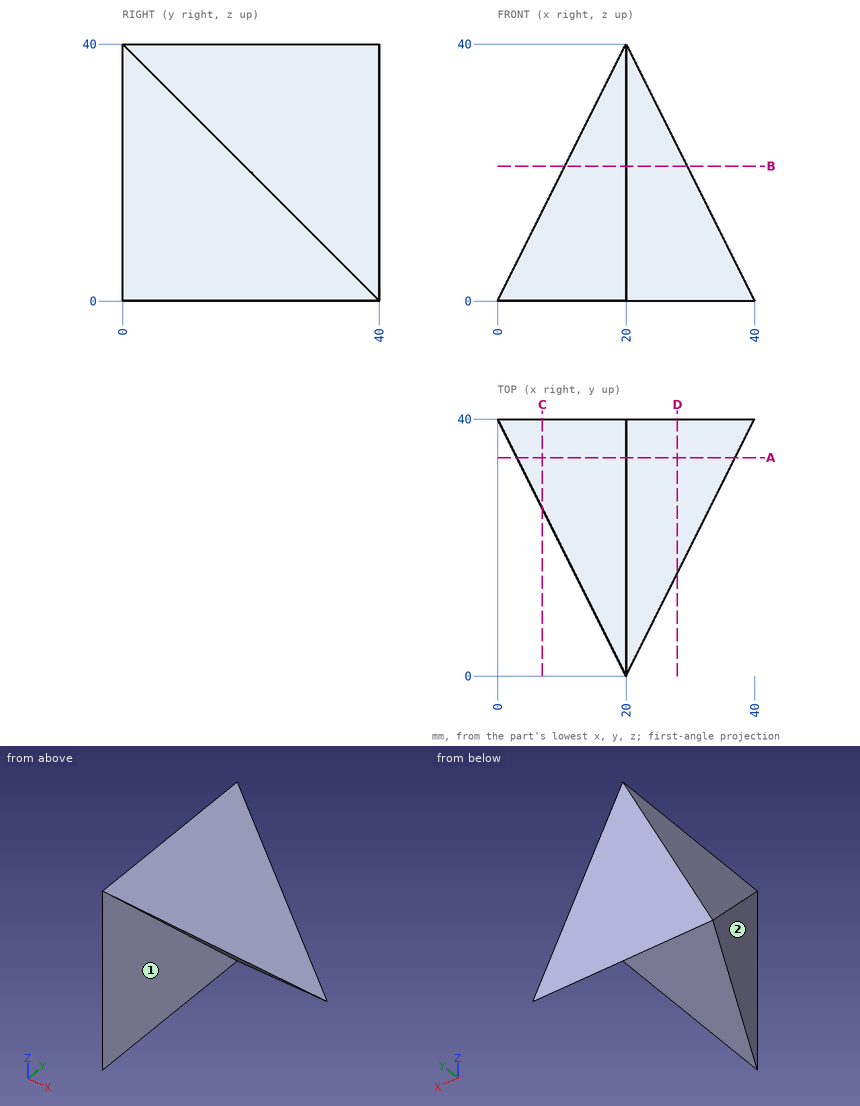
Print and shaded views of the part. All mm, measured from the part's lowest x, y and z. A direction names the side the tool comes from. Coordinates: 2 decimals unless noted, no trailing zeros. Order: outer loops, then holes, each group sorted by start corner. A loop starts at its lowest first (then second) coordinate and runs counter-clockwise, first axis right, second up.
(1) Slice it at C-C, the plane x = 7. Write the cut outline in (y, z).
Check sheet entries:
outline: (26, 0) - (40, 0) - (40, 14) - (26, 14) - close
(2) Slice it at A-A, the plane y = 34. Write the cut outline in (x, z), and give its area (3 significant figures).
Check sheet entries:
outline: (3, 0) - (20, 0) - (20, 6) - (37, 6) - (20, 40) - (3, 6) - close
area: 680 mm2
(3) Slice it at D-D, the plane x = 28. Write the cut outline in (y, z).
Check sheet entries:
outline: (16, 24) - (40, 0) - (40, 24) - close
(4) Probe L1, parallel to X at y = 4.5, z = 27.5; L2, parallel to Z at x = 29.5, y = 33; L3, parallel to Y at x = 26.5, z = 4.5. List the from-to ranges inside material, lowest first.
Check sheet entries:
L1: x = 17.75 to 20
L2: z = 7 to 21
L3: y = 35.5 to 40
(5) Tool access for the marked faces 1 and 2: list every direction of +Z, -Z, +X, -X, +Y, -Y with a clear straight run to the whole face (end or side of a thin tool).
Check sheet entries:
face 1: -Z, +X, -Y
face 2: +Z, -Z, -X, -Y
(6) Pin check, flat tips, straight feed: pin 1 Ø2 at (y, z) = (15, 6.5) entering from +X; pin 2 Ø8 at (y, z) = (32.5, 14.5) entering from +X; pin 3 Ø4 at (x, y) = (28, 12.5) entering from +Z. Stop position of each tip, or through.
Check sheet entries:
pin 1: stops at x = 20
pin 2: stops at x = 34.75
pin 3: stops at z = 28
(7) Slice it at B-B, the plane z = 21. Write the cut outline in (x, y), and give its area (3 significant figures).
Check sheet entries:
outline: (10.5, 19) - (20, 0) - (20, 19) - (29.5, 19) - (29.5, 40) - (10.5, 40) - close
area: 489 mm2
